For this review, take the finished solid that the model builds, in its own axes (mm). Face numbers are marked on the shaded views. A direction names the side the tool comes from. Give positions to 0.01 mm unless a question says otherwise; leave off trailing zeros. Order: outer loops, then holes, each group sorted by start corner. A loop starts at its lowest first (then second) coordinate and runs counter-clockwise, first axis right, second up. Notation, with made-up numbers: (-16.75, 64.25) - (14.25, 64.25) arc R16 cw to (14.25, 71.25) - close; hole circle Ø2 at (-40, 28.25). An arc over 180 degrees is marked (long way). One line per item, written item: value.
```python
from build123d import *

# Parameters (mm, degrees)
SKETCH1_R           = 1.6
BOSS_EXTRUDE1_DEPTH = 7.5
SKETCH2_W           = 29.4
SKETCH2_H           = 29.4
BOSS_EXTRUDE2_DEPTH = 7.5
SKETCH3_W           = 29.4
SKETCH3_H           = 31
SKETCH3_R           = 1.6
BOSS_EXTRUDE3_DEPTH = 7.5
FILLET1_R           = 5
FILLET2_R           = 2


with BuildPart() as part:
    # Sketch1 → Boss-Extrude1 (new body)
    with BuildSketch(Plane(origin=(0, 0, 0), x_dir=(1, 0, 0), z_dir=(0, 1, 0))):
        with BuildLine():
            Line((-5, 43.966606646), (-5, 44.520107817))
            ThreePointArc((-5, 44.520107817), (0, 44.8), (5, 44.520107817))
            Line((5, 44.520107817), (5, 43.966606646))
            ThreePointArc((5, 43.966606646), (31.289475068, 31.289475068), (43.966606646, 5))
            Line((43.966606646, 5), (44.520107817, 5))
            ThreePointArc((44.520107817, 5), (44.8, 0), (44.520107817, -5))
            Line((44.520107817, -5), (43.966606646, -5))
            ThreePointArc((43.966606646, -5), (31.289475068, -31.289475068), (5, -43.966606646))
            Line((5, -43.966606646), (5, -44.520107817))
            ThreePointArc((5, -44.520107817), (0, -44.8), (-5, -44.520107817))
            Line((-5, -44.520107817), (-5, -43.966606646))
            ThreePointArc((-5, -43.966606646), (-31.289475068, -31.289475068), (-43.966606646, -5))
            Line((-43.966606646, -5), (-44.520107817, -5))
            ThreePointArc((-44.520107817, -5), (-44.8, 0), (-44.520107817, 5))
            Line((-44.520107817, 5), (-43.966606646, 5))
            ThreePointArc((-43.966606646, 5), (-31.289475068, 31.289475068), (-5, 43.966606646))
        make_face()
        with Locations(Location((36.25, 0, 0), (0, 0, 270))):
            Circle(SKETCH1_R, mode=Mode.SUBTRACT)
        with Locations(Location((25.632620818, -25.632620818, 0), (0, 0, 270))):
            Circle(SKETCH1_R, mode=Mode.SUBTRACT)
        with Locations(Location((0, -36.25, 0), (0, 0, 270))):
            Circle(SKETCH1_R, mode=Mode.SUBTRACT)
        with Locations(Location((-25.632620818, -25.632620818, 0), (0, 0, 270))):
            Circle(SKETCH1_R, mode=Mode.SUBTRACT)
        with Locations(Location((-36.25, 0, 0), (0, 0, 270))):
            Circle(SKETCH1_R, mode=Mode.SUBTRACT)
        with Locations(Location((-25.632620818, 25.632620818, 0), (0, 0, 270))):
            Circle(SKETCH1_R, mode=Mode.SUBTRACT)
        with Locations(Location((0, 36.25, 0), (0, 0, 270))):
            Circle(SKETCH1_R, mode=Mode.SUBTRACT)
        with Locations(Location((25.632620818, 25.632620818, 0), (0, 0, 270))):
            Circle(SKETCH1_R, mode=Mode.SUBTRACT)
        with BuildLine():
            Line((33.430226046, 5), (36.586370413, 5))
            ThreePointArc((36.586370413, 5), (38.127746073, 5.725574218), (38.550739294, 7.375838926))
            ThreePointArc((38.550739294, 7.375838926), (36.262271651, 15.02032472), (32.474994896, 22.043983453))
            ThreePointArc((32.474994896, 22.043983453), (31.008980156, 22.911795444), (29.406004524, 22.334936712))
            Line((29.406004524, 22.334936712), (25.760059877, 18.688992065))
            Line((25.760059877, 18.688992065), (18.688992065, 25.760059877))
            Line((18.688992065, 25.760059877), (22.334936712, 29.406004524))
            ThreePointArc((22.334936712, 29.406004524), (22.911795444, 31.008980156), (22.043983453, 32.474994896))
            ThreePointArc((22.043983453, 32.474994896), (15.02032472, 36.262271651), (7.375838926, 38.550739294))
            ThreePointArc((7.375838926, 38.550739294), (5.725574218, 38.127746073), (5, 36.586370413))
            Line((5, 36.586370413), (5, 33.430226046))
            ThreePointArc((5, 33.430226046), (4.414213562, 32.016012484), (3, 31.430226046))
            Line((3, 31.430226046), (-3, 31.430226046))
            ThreePointArc((-3, 31.430226046), (-4.414213562, 32.016012484), (-5, 33.430226046))
            Line((-5, 33.430226046), (-5, 36.586370413))
            ThreePointArc((-5, 36.586370413), (-5.725574218, 38.127746073), (-7.375838926, 38.550739294))
            ThreePointArc((-7.375838926, 38.550739294), (-15.02032472, 36.262271651), (-22.043983453, 32.474994896))
            ThreePointArc((-22.043983453, 32.474994896), (-22.911795444, 31.008980156), (-22.334936712, 29.406004524))
            Line((-22.334936712, 29.406004524), (-18.688992065, 25.760059877))
            Line((-18.688992065, 25.760059877), (-25.760059877, 18.688992065))
            Line((-25.760059877, 18.688992065), (-29.406004524, 22.334936712))
            ThreePointArc((-29.406004524, 22.334936712), (-31.008980156, 22.911795444), (-32.474994896, 22.043983453))
            ThreePointArc((-32.474994896, 22.043983453), (-36.262271651, 15.02032472), (-38.550739294, 7.375838926))
            ThreePointArc((-38.550739294, 7.375838926), (-38.127746073, 5.725574218), (-36.586370413, 5))
            Line((-36.586370413, 5), (-33.430226046, 5))
            ThreePointArc((-33.430226046, 5), (-32.016012484, 4.414213562), (-31.430226046, 3))
            Line((-31.430226046, 3), (-31.430226046, -3))
            ThreePointArc((-31.430226046, -3), (-32.016012484, -4.414213562), (-33.430226046, -5))
            Line((-33.430226046, -5), (-36.586370413, -5))
            ThreePointArc((-36.586370413, -5), (-38.127746073, -5.725574218), (-38.550739294, -7.375838926))
            ThreePointArc((-38.550739294, -7.375838926), (-36.262271651, -15.02032472), (-32.474994896, -22.043983453))
            ThreePointArc((-32.474994896, -22.043983453), (-31.008980156, -22.911795444), (-29.406004524, -22.334936712))
            Line((-29.406004524, -22.334936712), (-25.760059877, -18.688992065))
            Line((-25.760059877, -18.688992065), (-18.688992065, -25.760059877))
            Line((-18.688992065, -25.760059877), (-22.334936712, -29.406004524))
            ThreePointArc((-22.334936712, -29.406004524), (-22.911795444, -31.008980156), (-22.043983453, -32.474994896))
            ThreePointArc((-22.043983453, -32.474994896), (-15.02032472, -36.262271651), (-7.375838926, -38.550739294))
            ThreePointArc((-7.375838926, -38.550739294), (-5.725574218, -38.127746073), (-5, -36.586370413))
            Line((-5, -36.586370413), (-5, -33.430226046))
            ThreePointArc((-5, -33.430226046), (-4.414213562, -32.016012484), (-3, -31.430226046))
            Line((-3, -31.430226046), (3, -31.430226046))
            ThreePointArc((3, -31.430226046), (4.414213562, -32.016012484), (5, -33.430226046))
            Line((5, -33.430226046), (5, -36.586370413))
            ThreePointArc((5, -36.586370413), (5.725574218, -38.127746073), (7.375838926, -38.550739294))
            ThreePointArc((7.375838926, -38.550739294), (15.02032472, -36.262271651), (22.043983453, -32.474994896))
            ThreePointArc((22.043983453, -32.474994896), (22.911795444, -31.008980156), (22.334936712, -29.406004524))
            Line((22.334936712, -29.406004524), (18.688992065, -25.760059877))
            Line((18.688992065, -25.760059877), (25.760059877, -18.688992065))
            Line((25.760059877, -18.688992065), (29.406004524, -22.334936712))
            ThreePointArc((29.406004524, -22.334936712), (31.008980156, -22.911795444), (32.474994896, -22.043983453))
            ThreePointArc((32.474994896, -22.043983453), (36.262271651, -15.02032472), (38.550739294, -7.375838926))
            ThreePointArc((38.550739294, -7.375838926), (38.127746073, -5.725574218), (36.586370413, -5))
            Line((36.586370413, -5), (33.430226046, -5))
            ThreePointArc((33.430226046, -5), (32.016012484, -4.414213562), (31.430226046, -3))
            Line((31.430226046, -3), (31.430226046, 3))
            ThreePointArc((31.430226046, 3), (32.016012484, 4.414213562), (33.430226046, 5))
        make_face(mode=Mode.SUBTRACT)
    extrude(amount=BOSS_EXTRUDE1_DEPTH)

    # Sketch2 → Boss-Extrude2 (add)
    with BuildSketch(Plane(origin=(0, 7.5, 0), x_dir=(1, 0, 0), z_dir=(0, 1, 0))):
        with BuildLine():
            Line((13.886291501, 22.2), (-13.886291501, 22.2))
            ThreePointArc((-13.886291501, 22.2), (-15.034341798, 22.428361402), (-16.007611845, 23.078679656))
            Line((-16.007611845, 23.078679656), (-18.688992065, 25.760059877))
            Line((-18.688992065, 25.760059877), (-25.760059877, 18.688992065))
            Line((-25.760059877, 18.688992065), (-23.078679656, 16.007611845))
            ThreePointArc((-23.078679656, 16.007611845), (-22.428361402, 15.034341798), (-22.2, 13.886291501))
            Line((-22.2, 13.886291501), (-22.2, -13.886291501))
            ThreePointArc((-22.2, -13.886291501), (-22.428361402, -15.034341798), (-23.078679656, -16.007611845))
            Line((-23.078679656, -16.007611845), (-25.760059877, -18.688992065))
            Line((-25.760059877, -18.688992065), (-18.688992065, -25.760059877))
            Line((-18.688992065, -25.760059877), (-16.007611845, -23.078679656))
            ThreePointArc((-16.007611845, -23.078679656), (-15.034341798, -22.428361402), (-13.886291501, -22.2))
            Line((-13.886291501, -22.2), (13.886291501, -22.2))
            ThreePointArc((13.886291501, -22.2), (15.034341798, -22.428361402), (16.007611845, -23.078679656))
            Line((16.007611845, -23.078679656), (18.688992065, -25.760059877))
            Line((18.688992065, -25.760059877), (25.760059877, -18.688992065))
            Line((25.760059877, -18.688992065), (23.078679656, -16.007611845))
            ThreePointArc((23.078679656, -16.007611845), (22.428361402, -15.034341798), (22.2, -13.886291501))
            Line((22.2, -13.886291501), (22.2, 13.886291501))
            ThreePointArc((22.2, 13.886291501), (22.428361402, 15.034341798), (23.078679656, 16.007611845))
            Line((23.078679656, 16.007611845), (25.760059877, 18.688992065))
            Line((25.760059877, 18.688992065), (18.688992065, 25.760059877))
            Line((18.688992065, 25.760059877), (16.007611845, 23.078679656))
            ThreePointArc((16.007611845, 23.078679656), (15.034341798, 22.428361402), (13.886291501, 22.2))
        make_face()
        Rectangle(SKETCH2_W, SKETCH2_H, mode=Mode.SUBTRACT)
    extrude(amount=-BOSS_EXTRUDE2_DEPTH)

    # Sketch3 → Boss-Extrude3 (add)
    with BuildSketch(Plane.XY.offset(-14.7)):
        with Locations((0, -10)):
            Rectangle(SKETCH3_W, SKETCH3_H)
        with Locations((-12, -21.5)):
            Circle(SKETCH3_R, mode=Mode.SUBTRACT)
        with Locations(Location((12, -21.5, 0), (0, 0, 180))):
            Circle(SKETCH3_R, mode=Mode.SUBTRACT)
    extrude(amount=-BOSS_EXTRUDE3_DEPTH)

    # Fillet1
    fillet1_edges = [part.edges().sort_by_distance(p)[0] for p in [
        (-14.7, 0, -18.45),
        (14.7, 0, -18.45),
    ]]
    fillet(fillet1_edges, radius=FILLET1_R)

    # Fillet2
    fillet2_edges = [part.edges().sort_by_distance(p)[0] for p in [
        (-14.7, -25.5, -18.45),
        (14.7, -25.5, -18.45),
    ]]
    fillet(fillet2_edges, radius=FILLET2_R)


solid = part.part
```
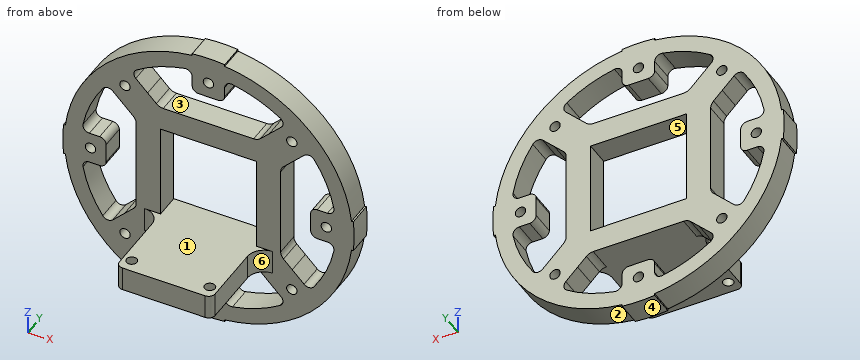
(1) Wall thickness on line 1 (X direction, y = 1.5, z = 9); line 2 (Y direction, x = 19.5, z = -4); line 3 (X direction, y = 4, z = 36): over which ranges is each line inside the solid? List them lowest first. Write a range as from..to.
Answers below:
line 1: x = -43.33..-38.2, -22.2..-14.7, 14.7..22.2, 38.2..43.33
line 2: y = 0..7.5
line 3: x = -25.73..-15.64, -5..-1.58, 1.58..5, 15.64..25.73
(2) Draft analysis for pull direction X (two halves, no side actions). For the marked faces 1, 2, 3 and 4, state which applies: pulls with the +X half, pulls with the -X half, needs draft (parallel to the pull), parting line crosses it, or undercut.
Answers below:
face 1: undercut
face 2: pulls with the +X half
face 3: undercut
face 4: parting line crosses it
(3) For P1, Ø1.6, axis at y = 4, z = 35, coming from the +X side; P2, Ø6, axis at y = 3, z = -3.5, coming from the +X side; P3, Ø1.6, axis at x = -34.5, y = 5, coming from the +Z side; P4, Ø3, axis at x = 0, z = 36.25, coming from the -Y side, all flat-tipped, find the tip position at first contact; note any pin that passes through.
Answers below:
P1: stops at x = 28.08
P2: stops at x = 44.8
P3: stops at z = 28.68
P4: passes through
(4) Take a section at C-C (y = -12). Write out the cut boundary in (x, z).
Answers below:
outline: (-14.7, -22.2) - (14.7, -22.2) - (14.7, -14.7) - (-14.7, -14.7) - close
(5) Machinability: for the marked faces 5 and 6, which of the approach directions +Z, -Z, +X, -X, +Y, -Y give a long, thin tool a straight path to every point of the face, cutting with its end or side? Answer none if there is none.
Answers below:
face 5: +Y, -Y
face 6: +Z, -Z, +X, -Y
(6) Take a section at A-A (z = 0). Write out the cut boundary in (x, y).
Answers below:
outline: (-44.8, 0) - (-37.85, 0) - (-37.85, 7.5) - (-44.8, 7.5) - close; (-34.65, 0) - (-31.43, 0) - (-31.43, 7.5) - (-34.65, 7.5) - close; (-22.2, 0) - (-14.7, 0) - (-14.7, 7.5) - (-22.2, 7.5) - close; (14.7, 0) - (22.2, 0) - (22.2, 7.5) - (14.7, 7.5) - close; (31.43, 0) - (34.65, 0) - (34.65, 7.5) - (31.43, 7.5) - close; (37.85, 0) - (44.8, 0) - (44.8, 7.5) - (37.85, 7.5) - close
(7) Take a section at B-B (x = 0). Write out the cut boundary in (y, z), then the cut area to 3 significant figures.
Answers below:
outline: (-25.5, -22.2) - (7.5, -22.2) - (7.5, -14.7) - (-25.5, -14.7) - close; (0, -44.8) - (7.5, -44.8) - (7.5, -37.85) - (0, -37.85) - close; (0, -34.65) - (7.5, -34.65) - (7.5, -31.43) - (0, -31.43) - close; (0, 14.7) - (7.5, 14.7) - (7.5, 22.2) - (0, 22.2) - close; (0, 31.43) - (7.5, 31.43) - (7.5, 34.65) - (0, 34.65) - close; (0, 37.85) - (7.5, 37.85) - (7.5, 44.8) - (0, 44.8) - close
area: 456 mm^2
(8) Take a section at D-D (y = 2). Give the number of separate pieces and of enclosed holes in the cut face, then the cut area to 3 significant figures.
Answers below:
separate pieces: 1
enclosed holes: 13
area: 3,110 mm^2
